Read the model definition and answer for the solid it produces. Units are mm, in the model's axes. A direction names the side the tool comes from. Coordinates: 2 decimals unless noted, no trailing zeros. Write each loop counter-clockwise with the first axis right and the second up, starting at its lowest first coordinate (ties: lowest second). Pieces come first, ordered by that corner, then holes.
Item 1: Straight lines are drawn through the part: probe 1 along Z at (x, y) = (-2.25, 2.2) (3 decimals); probe 2 along X at (y, z) = (2.05, -0.7); probe 3 along Z at (x, y) = (3.75, 2). For each, find the intervals that lie inside material, in ascending order.
Item 2: Section B-B (x = 0.75) is taken. Give the vertices of the cut face in (y, z) (3 decimals).
Item 3: A tool of negligible diameter and unlimited length cuts with its end or side. For faces 1 (the face through (0, 2, -1.925)), 2 (the face through (-5.125, 1.734, -0.042)), 3 (the face through (5.125, 1.734, 0.042)), from which of +Z, -Z, +X, -X, +Y, -Y can it reach the whole face along a straight path? Write none if from no direction.
Item 4: Section A-A (z = 0) is taken. Give the vertices of the cut face in (x, y) (3 decimals), then the cut area to 3 significant figures.
Item 5: Section C-C (y = 1.95) is taken. Give the vertices of the cut face in (x, z) (3 decimals).
Item 6: Each of these flat-tipped pins is pushed along its axis until it touches: P1, Ø1.2, axis at x = 0, y = 2, coming from the -Z side (3 decimals); P2, Ø0.8, axis at x = -1, y = 2, coming from the +Z side (3 decimals). Where does it stop, or does it pass through?
Item 7: Section D-D (y = 0.3) is taken. Give the vertices of the cut face in (x, z) (3 decimals).
from build123d import *

# Parameters (mm, degrees)
BOSS_EXTRUDE1_DEPTH = 0.5
BOSS_EXTRUDE2_DEPTH = 2.5
FILLET1_R           = 0.5
FILLET3_R           = 0.5


with BuildPart() as part:
    # Sketch1 → Boss-Extrude1 (new body)
    with BuildSketch(Plane(origin=(0, 0, 0), x_dir=(1, 0, 0), z_dir=(0, 1, 0))):
        with BuildLine():
            Line((-3.2, 2.325), (3.2, 2.325))
            ThreePointArc((3.2, 2.325), (5.525, 0), (3.2, -2.325))
            Line((3.2, -2.325), (-3.2, -2.325))
            ThreePointArc((-3.2, -2.325), (-5.525, 0), (-3.2, 2.325))
        make_face()
    extrude(amount=BOSS_EXTRUDE1_DEPTH)

    # Sketch2 → Boss-Extrude2 (add)
    with BuildSketch(Plane(origin=(0, 0.5, 0), x_dir=(1, 0, 0), z_dir=(0, 1, 0))):
        with BuildLine():
            Line((-3.2, -1.925), (3.2, -1.925))
            ThreePointArc((3.2, -1.925), (5.125, 0), (3.2, 1.925))
            Line((3.2, 1.925), (-3.2, 1.925))
            ThreePointArc((-3.2, 1.925), (-5.125, 0), (-3.2, -1.925))
        make_face()
    extrude(amount=BOSS_EXTRUDE2_DEPTH)

    # Fillet1
    # the kernel refuses this fillet: 0.5 mm, written as the material it adds along each edge
    with BuildSketch(Plane(origin=(-3.2, 0.5, 0), x_dir=(0, 0, -1), z_dir=(1, 0, 0))) as fillet1_piece_1:
        with BuildLine():
            CenterArc((2.425, 0.489897949), FILLET1_R, 180, 78.463040967)
            Line((1.925, 0.489897949), (1.915, 0.489897949))
            Line((1.915, 0.489897949), (1.915, 0))
            Line((1.915, 0), (1.925, -0.01))
            ThreePointArc((1.925, -0.01), (2.125, -0.01), (2.323, -0.009797959))
            Line((2.323, -0.009797959), (2.325, 0))
        make_face()
    revolve(axis=Axis((-3.2, 0.5, 0), (0, 1, 0)), revolution_arc=180)
    with BuildSketch(Plane(origin=(-3.2, 0.5, 1.925), x_dir=(0, 1.5665246877455952e-12, 1.0), z_dir=(1, 0, 0)), Plane(origin=(3.2, 0.5, -1.925), x_dir=(0, 1.5665246877455952e-12, -1.0), z_dir=(-1, 0, 0))) as fillet1_piece_2:
        with BuildLine():
            CenterArc((0.5, -0.489897949), FILLET1_R, 101.536959033, 78.463040967)
            Line((0, -0.489897949), (-0.01, -0.489897949))
            Line((-0.01, -0.489897949), (-0.01, 0))
            Line((-0.01, 0), (0, 0.01))
            ThreePointArc((0, 0.01), (0.2, 0.01), (0.398, 0.009797959))
            Line((0.398, 0.009797959), (0.4, 0))
        make_face()
    extrude(amount=6.4)
    with BuildSketch(Plane(origin=(3.2, 0.5, 0), x_dir=(0, 0, 1), z_dir=(-1, 0, 0))) as fillet1_piece_3:
        with BuildLine():
            CenterArc((2.425, 0.489897949), FILLET1_R, 180, 78.463040967)
            Line((1.925, 0.489897949), (1.915, 0.489897949))
            Line((1.915, 0.489897949), (1.915, 0))
            Line((1.915, 0), (1.925, -0.01))
            ThreePointArc((1.925, -0.01), (2.125, -0.01), (2.323, -0.009797959))
            Line((2.323, -0.009797959), (2.325, 0))
        make_face()
    revolve(axis=Axis((3.2, 0.5, 0), (0, 1, 0)), revolution_arc=180)

    # Fillet3
    fillet3_edges = [part.edges().sort_by_distance(p)[0] for p in [
        (-5.125, 3, 0),
        (0, 3, 1.925),
        (5.125, 3, 0),
        (0, 3, -1.925),
    ]]
    fillet(fillet3_edges, radius=FILLET3_R)


solid = part.part
Established:
1. probe 1: z = -1.925 to 1.925
1. probe 2: x = -4.99 to 4.99
1. probe 3: z = -1.84 to 1.84
2. outline: (0, -2.325) - (0.5, -2.325) arc R0.5 cw to (0.99, -1.925) - (2.5, -1.925) arc R0.5 ccw to (3, -1.425) - (3, 1.425) arc R0.5 ccw to (2.5, 1.925) - (0.99, 1.925) arc R0.5 cw to (0.5, 2.325) - (0, 2.325) - close
3. face 1: -Z, +X, -X, +Y
3. face 2: -X, +Y
3. face 3: +X, +Y
4. outline: (-5.525, 0) - (5.525, 0) - (5.525, 0.5) arc R0.5 cw to (5.125, 0.99) - (5.125, 2.5) arc R0.5 ccw to (4.625, 3) - (-4.625, 3) arc R0.5 ccw to (-5.125, 2.5) - (-5.125, 0.99) arc R0.5 cw to (-5.525, 0.5) - close
4. area: 31.1 mm2
5. outline: (-3.2, -1.925) - (3.2, -1.925) arc R1.925 ccw to (3.2, 1.925) - (-3.2, 1.925) arc R1.925 ccw to start
6. P1: stops at z = -1.925
6. P2: stops at z = 1.925
7. outline: (-3.2, -2.325) - (3.2, -2.325) arc R2.325 ccw to (3.2, 2.325) - (-3.2, 2.325) arc R2.325 ccw to start
